```python
from build123d import *

# Parameters (mm, degrees)
REVOLVE2_ANGLE     = 360
CUT_EXTRUDE2_DEPTH = 1.925
SKETCH6_R          = 1.732050808
CUT_EXTRUDE3_DEPTH = 1.925
CUT_EXTRUDE3_DRAFT = -45


with BuildPart() as part:
    # Sketch10 → Revolve3 (revolve)
    with BuildSketch(Plane(origin=(0, 0, 0), x_dir=(0, 0, -1), z_dir=(1, 0, 0))):
        Polygon((32.15, 2.5), (32.75, 1.9), (32.75, 0), (2.75, 0), (2.75, 2.5), align=None)
    revolve(axis=Axis((0, 0, 0), (0, 0, -1)))

    # Sketch7 → Revolve2 (revolve, symmetric)
    with BuildSketch(Plane(origin=(0, 0, 0), x_dir=(0, 0, -1), z_dir=(1, 0, 0))) as revolve2_sk:
        with BuildLine():
            Line((2.3375, 4.75), (2.75, 4.75))
            Line((2.75, 4.75), (2.75, 0))
            Line((2.75, 0), (0, 0))
            Line((0, 0), (0, 2.5))
            ThreePointArc((0, 2.5), (0.991875183, 3.808753282), (2.3375, 4.75))
        make_face()
    revolve(axis=Axis((0, 0, 0), (0, 0, -1)), revolution_arc=REVOLVE2_ANGLE / 2)
    revolve(revolve2_sk.sketch, axis=Axis((0, 0, 0), (0, 0, 1)), revolution_arc=REVOLVE2_ANGLE / 2)

    # Sketch5 → Cut-Extrude2 (cut)
    with BuildSketch(Plane.XY):
        Polygon((1.5, -0.866025404), (1.5, 0.866025404), (0, 1.732050808), (-1.5, 0.866025404), (-1.5, -0.866025404), (0, -1.732050808), align=None)
    extrude(amount=-CUT_EXTRUDE2_DEPTH, mode=Mode.SUBTRACT)


with BuildPart() as cut_extrude3_tool:
    # Sketch6 → Cut-Extrude3 (with draft: the straight prism first)
    with BuildSketch(Plane.XY):
        Circle(SKETCH6_R)
    extrude(amount=-CUT_EXTRUDE3_DEPTH)
    # Cut-Extrude3: the draft: its side faces are tilted about the plane it starts from
    cut_extrude3_sides = [cut_extrude3_tool.faces().sort_by_distance(p)[0] for p in [
        (-1.732050808, 0, -0.9625),
    ]]
    draft(cut_extrude3_sides, Plane.XY, CUT_EXTRUDE3_DRAFT)


with BuildPart() as part_1:
    add(part.part)

    # Cut-Extrude3: cut by cut_extrude3_tool
    add(cut_extrude3_tool.part, mode=Mode.SUBTRACT)


solid = part_1.part
```
Read the model definition and answer for the solid it produces. Units are mm, in the model's axes. A direction names the side the tool comes from. Round coordinates to 2 decimals unless told otherwise and drop trailing zeros. Write each loop counter-clockwise with the first axis right and the second up, starting at its lowest first coordinate (ties: lowest second). Pieces come first, ordered by that corner, then holes. Notation, with made-up numbers: (35, 30) - (93, 30) arc R12 ccw to (93, 38) - close; hole circle Ø10 at (-26.75, -4.75). An arc over 180 degrees is marked (long way). Use CSV: the item, a comma, the result in double quotes.
Q1. Straight lines are drawn through the part: line 1 along Z through (x, y) = (-1, 0.5) (3 decimals); line 2 along Y through (x, z) = (-1, -8); line 3 along X through (y, z) = (-0.5, -23.5). For each, find the intervals that lie inside material, in ascending order.
Values:
line 1,"z = -32.75 to -1.925"
line 2,"y = -2.29 to 2.29"
line 3,"x = -2.45 to 2.45"
Q2. Find section C-C, the plane x = -3.25. Write down the section's boundary in (y, z), then the cut area to 3 significant figures.
Values:
outline,"(-3.46, -2.75) - (3.46, -2.75) - (3.46, -2.34) arc R4.17 ccw to (-3.46, -2.34) - close"
area,"11.9 mm²"
Q3. A tool of negligible diameter and unlimited length cuts with its end or side. For faces 1 (the flat face through (0, 0, -32.75)), 2 (the conical face through (0.8, -1.41, -0.11)), from which of +Z, -Z, +X, -X, +Y, -Y can it reach the whole face along a straight path? Write none if from no direction.
Values:
face 1,"-Z, +X, -X, +Y, -Y"
face 2,"+Z"
Q4. Find section D-D, the plane y = -4. Write down the section's boundary in (x, z), then the cut area to 3 significant figures.
Values:
outline,"(-2.56, -2.75) - (2.56, -2.75) - (2.56, -2.34) arc R3.46 ccw to (-2.56, -2.34) - close"
area,"6.14 mm²"
Q5. Find section B-B, the plane z = -28.5. Write down the section's boundary in (x, y), then the cut area to 3 significant figures.
Values:
outline,"circle Ø5 at (0, 0)"
area,"19.6 mm²"
Q6. Each of these flat-tipped pins is pushed along its axis until it touches: pin 1 Ø3 at (y, z) = (-2, -7) entering from -X; pin 2 Ø1.5 at (y, z) = (-1, -16.5) entering from +X; pin 3 Ø0.5 at (y, z) = (0, -1.5) entering from +X. Where does it stop, or does it pass through?
Values:
pin 1,"stops at x = -2.45"
pin 2,"stops at x = 2.49"
pin 3,"stops at x = 4.41"
Q7. Determine the mould class of faces 3 (the flat face through (2, 2, -2.75)), 4 (the flat face through (-1.5, 0, -1)), 5 (the cylindrical face through (-2.44, -0.54, -17.66)) for opening direction Y: +Y half, -Y half, draft (parallel to the pull), parting line (faces both ways), or undercut.
Values:
face 3,"draft"
face 4,"undercut"
face 5,"parting line"
